The model under review builds one solid part; all positions refer to its coordinate system, in mm. Face numbers are marked on the shaded views. A direction names the side the tool comes from. Give positions to 0.01 mm unless a question says otherwise; leave off trailing zeros. Order: outer loops, then holes, each group sorted by start corner. A loop starts at its lowest first (then second) coordinate and runs counter-clockwise, first axis right, second up.
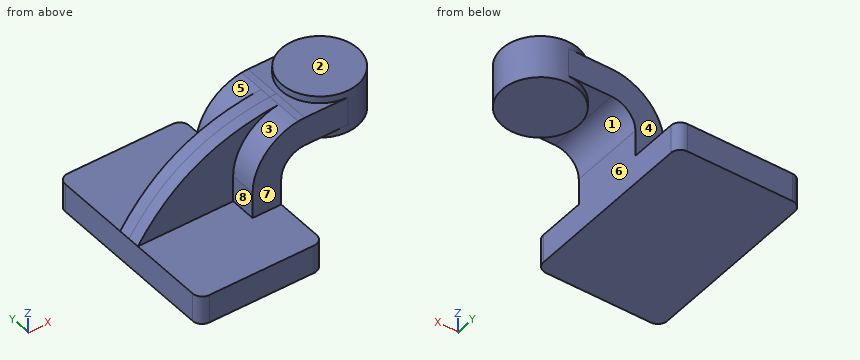
```python
from build123d import *

# Parameters (mm, degrees)
F1_DEPTH = 63.5
F0_W     = 25.4
F0_H     = 19.05
F2_DEPTH = 25.4
F3_DEPTH = 7.9375
F5_R     = 6.35


# Not quite as in the source:
# - a feature names something its author has since deleted; it is built from what else it names


with BuildPart() as f1:
    # F0 (on Front) → F1 (new body, symmetric)
    with BuildSketch(Plane.XZ):
        Polygon((22.225, 9.525), (-41.275, 9.525), (-41.275, -9.525), (41.275, -9.525), (41.275, 9.525), align=None)
    extrude(amount=F1_DEPTH, both=True)



with BuildPart() as f2:
    # F0 (on Front) → F2 (new body, symmetric)
    with BuildSketch(Plane.XZ):
        with BuildLine():
            Line((22.225, 27.0517572581), (22.225, 9.525))
            Line((22.225, 9.525), (41.275, 9.525))
            Line((41.275, 9.525), (41.275, 27.0517572581))
            ThreePointArc((41.275, 27.0517572581), (45.8699924784, 38.2221223064), (56.9949439764, 42.926))
            Line((56.9949439764, 42.926), (60.325, 42.926))
            Line((60.325, 42.926), (60.325, 61.976))
            Line((60.325, 61.976), (56.9200132545, 61.976))
            add(Edge.make_bspline(
                [(52.6300958014, 61.6830450054), (54.0440250085, 61.794890112), (55.4739013545, 61.892529432), (56.9200132545, 61.976)],
                knots=[107.8358858106, 107.8358858106, 107.8358858106, 107.8358858106, 111.3255048452, 111.3255048452, 111.3255048452, 111.3255048452], degree=3))
            ThreePointArc((52.6300958014, 61.6830450054), (30.9048739845, 50.0940875532), (22.225, 27.0517572581))
        make_face()
        with Locations((73.025, 52.451)):
            Rectangle(F0_W, F0_H)
    extrude(amount=F2_DEPTH, both=True)


with BuildPart() as f1_1:
    add(f1.part)

    add(f2.part)  # F3 merges F2
    # F0 (on Front) → F3 (join, symmetric)
    with BuildSketch(Plane.XZ):
        with BuildLine():
            add(Edge.make_bspline(
                [(-41.275, 9.525), (-19.5277563413, 41.2050885172), (8.9369857489, 58.2268178266), (52.6300958014, 61.6830450054)],
                knots=[0, 0, 0, 0, 107.8358858106, 107.8358858106, 107.8358858106, 107.8358858106], degree=3))
            Line((-41.275, 9.525), (22.225, 9.525))
            Line((22.225, 9.525), (22.225, 27.0517572581))
            ThreePointArc((22.225, 27.0517572581), (30.9048739845, 50.0940875532), (52.6300958014, 61.6830450054))
        make_face()
    extrude(amount=F3_DEPTH, both=True)

    # F0 (on Front) → F4 (revolve)
    with BuildSketch(Plane.XZ):
        Polygon((85.725, 66.675), (85.725, 61.976), (85.725, 42.926), (85.725, 38.1), (111.125, 38.1), (111.125, 66.675), align=None)
    revolve(axis=Axis((85.725, 0, 52.3875), (0, 0, -1)))

    # F5
    f5_edges = [f1_1.edges().sort_by_distance(p)[0] for p in [
        (-41.275, -63.5, 0),
        (41.275, -63.5, 0),
        (41.275, 63.5, 0),
        (-41.275, 63.5, 0),
    ]]
    fillet(f5_edges, radius=F5_R)


solid = f1_1.part
```
1. Draft analysis for pull direction X (two halves, no side actions). For the marked faces 1, 2 and 3, state which applies: pulls with the +X half, pulls with the -X half, needs draft (parallel to the pull), parting line crosses it, or undercut.
2. Take a section at C-C (y = 30). Write out the cut boundary in (x, z) (3 decimals), and give its area (3 significant figures).
3. To check wall thickness, follow line 1 (Y direction, x = 9, z = 32.5); line 2 (Z direction, x = 24, y = 32) (3 decimals); line 3 (Y direction, x = 72.5, z = 47). State the ranges of each line that lie inside material, in increasing order.
4. Insertion check: pin 1 (18.5 mm diameter, centred on y = 19.5, z = 11.5, fed in from +X) (3 decimals); pin 2 (1 mm diameter, centred on x = 38, z = 21.5, fed in from +Y); pin 3 (12 mm diameter, centred on y = 6.5, z = 44.5, fed in from -X). Each pin has a flat end and moves straight along its axis. Give the tip position at first contact, or say it passes through.
5. Take a section at B-B (x = 66.5). Write out the cut boundary in (y, z) (3 decimals), and give its area (3 significant figures).
6. Take a section at A-A (z = 3.5). Write out the cut boundary in (x, y) (3 decimals), and give its area (3 significant figures).
7. For the marked faces 4, 5, 6, 7 and 8, list the 3-axis set-ups (+Z, -Z, +X, -X, +Y, -Y) from which the entire face can be reached by the end or side of a thin tool; tool diameter is ignored.
Answer:
1. face 1: undercut
1. face 2: needs draft
1. face 3: pulls with the -X half
2. outline: (-41.275, -9.525) - (41.275, -9.525) - (41.275, 9.525) - (-41.275, 9.525) - close
2. area: 1,570 mm2
3. line 1: y = -7.94 to 7.94
3. line 2: z = -9.525 to 9.525
3. line 3: y = -25.4 to 25.4
4. pin 1: stops at x = 41.275
4. pin 2: stops at y = 25.4
4. pin 3: stops at x = -14.24
5. outline: (-25.4, 42.926) - (-16.6, 42.926) - (-16.6, 38.1) - (16.6, 38.1) - (16.6, 42.926) - (25.4, 42.926) - (25.4, 61.976) - (16.6, 61.976) - (16.6, 66.675) - (-16.6, 66.675) - (-16.6, 61.976) - (-25.4, 61.976) - close
5. area: 1,280 mm2
6. outline: (-41.275, -57.15) arc R6.35 ccw to (-34.925, -63.5) - (34.925, -63.5) arc R6.35 ccw to (41.275, -57.15) - (41.275, 57.15) arc R6.35 ccw to (34.925, 63.5) - (-34.925, 63.5) arc R6.35 ccw to (-41.275, 57.15) - close
6. area: 10,400 mm2
7. face 4: +Z, +X, -X, +Y
7. face 5: +Z, -X, +Y
7. face 6: -Z, +X, +Y, -Y
7. face 7: +Z, +X, -X, -Y
7. face 8: +Z, -X, -Y
